Geometry check sheet. Reference: drawing and pictorial views, mm from the part's lowest x, y, z. A direction names the side the tool comes from. Round coordinates to 2 decimals unless told otherwise and drop trailing zeros. Order: outer loops, then holes, each group sorted by start corner. A loop starts at its lowest first (then second) coordinate and runs counter-clockwise, first axis right, second up. Notation, with made-up numbers: (19, -2.75) -> (65, -2.75) arc R13 cw to (65, 6.25) -> close; hole circle Ø4 at (8.5, 81.25). An arc over 180 degrees is marked (long way). Put each result on its own line as item: value.
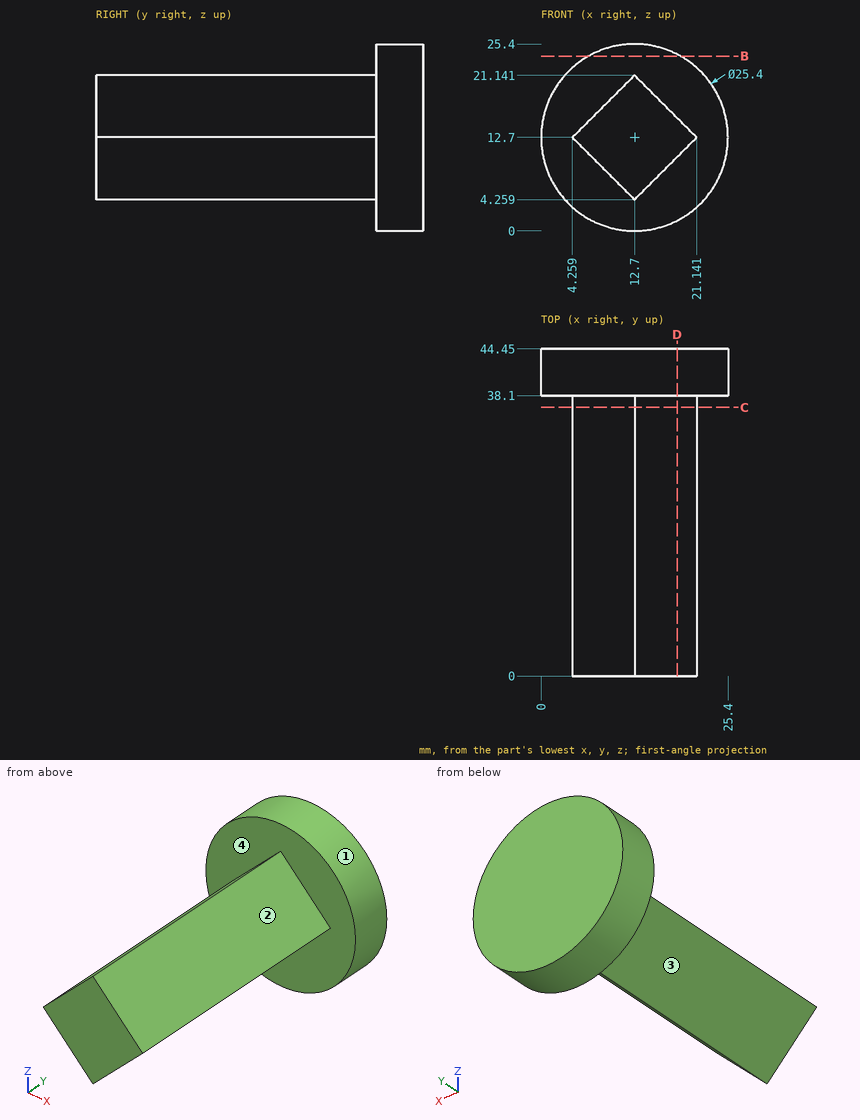
Item 1: Material ranges on line 1 along Y through (x, z) = (16.25, 19); line 2 along Z through (x, y) = (12.75, 40); line 3 along X through (y, z) = (39, 15.5), recorded low to high.
Geometry check:
line 1: 38.1 to 44.45
line 2: 0 to 25.4
line 3: 0.31 to 25.09
Item 2: Tool access check on the marked faces 1, 2, 3 and 4. Record the directions out of +Z, -Z, +X, -X, +Y, -Y that give a thin tool (end or side, any length) a straight path to the whole face; none if there is none.
Geometry check:
face 1: +Y, -Y
face 2: +Z, +X, -Y
face 3: -Z, -X, -Y
face 4: -Y
Item 3: Depth check by flat-ended pin: pin 1 Ø8 at (y, z) = (30.5, 19) entering from -X; pin 2 Ø12 at (y, z) = (14, 5.5) entering from +X; pin 3 Ø8 at (y, z) = (20.5, 3) entering from -X. Enter the tip coordinate at first touch or a pass-through.
Geometry check:
pin 1: x = 6.56
pin 2: x = 19.94
pin 3: x = 9.96
Item 4: Sectioned sample at D-D, the plane x = 18.5. Record the boundary of the cut face in (y, z), then the cut area to 3 significant figures.
Geometry check:
outline: (0, 10.06) -> (38.1, 10.06) -> (38.1, 1.4) -> (44.45, 1.4) -> (44.45, 24) -> (38.1, 24) -> (38.1, 15.34) -> (0, 15.34) -> close
area: 345 mm2
Item 5: Sectioned sample at C-C, the plane y = 36.5. Record the boundary of the cut face in (x, z).
Geometry check:
outline: (4.26, 12.7) -> (12.7, 4.26) -> (21.14, 12.7) -> (12.7, 21.14) -> close
Item 6: Sectioned sample at B-B, the plane z = 23.75. Record the boundary of the cut face in (x, y).
Geometry check:
outline: (6.44, 38.1) -> (18.96, 38.1) -> (18.96, 44.45) -> (6.44, 44.45) -> close
